Source: CAD feature listing. Evaluate the final solid. Frame: model axes, mm. Round coordinates to 2 decimals unless told otherwise and drop trailing zeros. Write each loop counter-clockwise with the first axis right and the second up, starting at its lowest first coordinate (ties: lowest second). Pieces come first, ordered by that corner, then holes. Notation, with made-up numbers: M 67.25,33 L 111.25,33 A18 cw 111.25,46 Z; hole C -34.5,55 d9. An arc over 180 degrees is marked long. Answer in a Markdown table with one row per item. Add a question column.
Item 1: Contact query for flat-ended pins moving along their axis: pin 1 (3 mm diameter, centred on x = 58, y = 13, fed in from -Z); pin 2 (6 mm diameter, centred on x = 58, y = -13, fed in from -Z). Output: stop coordinate, or through.
Item 2: Cut plane C-C on y = -13. Return loops of the section in (x, z), and give its area (3 significant figures).
Item 3: Cut plane B-B on x = 58. Return loops of the section in (y, z), and give its area (3 significant figures).
Item 4: Material intervals for probe 1 along Y at (x, z) = (58, 1.9); probe 2 along X at (y, z) = (16.5, 1.3); probe 3 along Y at (x, z) = (35, 4.5), sorted ascending.
Item 5: Mould query, pull axis Y, two halves, no side actions, for faces 1 (the face through (-1, 0, 0)), 2 (the face through (-55.69, 12.04, 2.54)), 3 (the face through (-55, -20, 2)), 4 (the face through (-55.69, -13.96, 2.54)). Classes: released by +Y, released by -Y, zero draft, split by the parting line, or undercut.
Item 6: Cut plane D-D on x = -2. Return loops of the section in (y, z), and give its area (3 significant figures).
Item 7: Cut plane A-A on z = 3.7. Return loops of the section in (x, y).
from build123d import *

# Parameters (mm, degrees)
F1_DEPTH = 5
F2_R     = 2.5
F3_DEPTH = 5.001


with BuildPart() as f1:
    # F0 (on Top) → F1 (new body)
    with BuildSketch(Plane.XY):
        with BuildLine():
            Line((-45, 20), (-65, 20))
            Line((-65, 20), (-65, -20))
            Line((-65, -20), (-45, -20))
            ThreePointArc((-45, -20), (0, -9), (45, -20))
            Line((45, -20), (65, -20))
            Line((65, -20), (65, 20))
            Line((65, 20), (45, 20))
            ThreePointArc((45, 20), (0, 9), (-45, 20))
        make_face()
    extrude(amount=F1_DEPTH)

    # F2 (on face) → F3 (cut, through all)
    with BuildSketch(Plane.XY.offset(5)):
        with Locations((-58, 13)):
            Circle(F2_R)
        with Locations((-58, -13)):
            Circle(F2_R)
        with Locations((58, 13)):
            Circle(F2_R)
        with Locations((58, -13)):
            Circle(F2_R)
    extrude(amount=-F3_DEPTH, mode=Mode.SUBTRACT)


solid = f1.part
Results below:
| question | item | result |
|---|---|---|
| 1 | pin 1 | through |
| 1 | pin 2 | z = 0 |
| 2 | outline | M -65,0 L -60.5,0 L -60.5,5 L -65,5 Z; M -55.5,0 L -27.65,0 L -27.65,5 L -55.5,5 Z; M 27.65,0 L 55.5,0 L 55.5,5 L 27.65,5 Z; M 60.5,0 L 65,0 L 65,5 L 60.5,5 Z |
| 2 | area | 324 mm2 |
| 3 | outline | M -20,0 L -15.5,0 L -15.5,5 L -20,5 Z; M -10.5,0 L 10.5,0 L 10.5,5 L -10.5,5 Z; M 15.5,0 L 20,0 L 20,5 L 15.5,5 Z |
| 3 | area | 150 mm2 |
| 4 | probe 1 | -20 to -15.5, -10.5 to 10.5, 15.5 to 20 |
| 4 | probe 2 | -65 to -37.51, 37.51 to 65 |
| 4 | probe 3 | -15.5 to 15.5 |
| 5 | face 1 | zero draft |
| 5 | face 2 | undercut |
| 5 | face 3 | released by -Y |
| 5 | face 4 | undercut |
| 6 | outline | M -9.02,0 L 9.02,0 L 9.02,5 L -9.02,5 Z |
| 6 | area | 90.2 mm2 |
| 7 | outline | M -65,-20 L -45,-20 A97.55 cw 45,-20 L 65,-20 L 65,20 L 45,20 A97.55 cw -45,20 L -65,20 Z; hole C -58,-13 d5; hole C -58,13 d5; hole C 58,-13 d5; hole C 58,13 d5 |
